from build123d import *

# Parameters (mm, degrees)
SKETCH2_W                      = 38.1
SKETCH2_H                      = 69.85
BOSS_EXTRUDE1_DEPTH            = 4.7625
FILLET1_R                      = 6.35
F_4_CLEARANCE_HOLE1_D          = 2.9464
BOSS_EXTRUDE2_DEPTH            = 9.525
F_8_32_TAPPED_HOLE1_AT_2_COUNT = 2
F_8_32_TAPPED_HOLE1_AT_2_PITCH = 28.575
F_8_32_TAPPED_HOLE1_AT_3_COUNT = 2
F_8_32_TAPPED_HOLE1_AT_3_PITCH = 28.575
SKETCH12_W                     = 19.05
SKETCH12_H                     = 44.45
CUT_EXTRUDE1_DEPTH             = 47.198333888
FILLET2_R                      = 3.175
F_8_32_TAPPED_HOLE2_D          = 3.4544


with BuildPart() as part:
    # Sketch2 → Boss-Extrude1 (new, symmetric)
    with BuildSketch(Plane.XY):
        Rectangle(SKETCH2_W, SKETCH2_H)
    extrude(amount=BOSS_EXTRUDE1_DEPTH, both=True)

    # Fillet1
    fillet1_edges = [part.edges().sort_by_distance(p)[0] for p in [
        (19.05, -34.925, 0),
        (-19.05, -34.925, 0),
        (-19.05, 34.925, 0),
        (19.05, 34.925, 0),
    ]]
    fillet(fillet1_edges, radius=FILLET1_R)

    # #4 Clearance Hole1 (through all)
    with Locations(Plane.XY.offset(4.7625)):
        with Locations((0, 29.21), (-15.24, 27.94), (15.24, 27.94), (-15.24, -27.94), (15.24, -27.94), (-16.51, 17.78), (-16.51, -12.7), (16.51, 17.78), (16.51, -12.7), (0, -29.21)):
            Hole(F_4_CLEARANCE_HOLE1_D / 2)

    # Sketch6 → Boss-Extrude2 (add)
    with BuildSketch(Plane(origin=(0, 0, -4.7625), x_dir=(-1, 0, 0), z_dir=(0, 0, -1))):
        with BuildLine():
            Line((-28.702, -34.925), (-12.7, -34.925))
            ThreePointArc((-12.7, -34.925), (-17.190128061, -33.065128061), (-19.05, -28.575))
            Line((-19.05, -28.575), (-19.05, 28.575))
            ThreePointArc((-19.05, 28.575), (-17.190128061, 33.065128061), (-12.7, 34.925))
            Line((-12.7, 34.925), (-28.702, 34.925))
            Line((-28.702, 34.925), (-28.702, -34.925))
        make_face()
        with BuildLine():
            Line((28.702, -34.925), (28.702, 34.925))
            Line((28.702, 34.925), (12.7, 34.925))
            ThreePointArc((12.7, 34.925), (17.190128061, 33.065128061), (19.05, 28.575))
            Line((19.05, 28.575), (19.05, -28.575))
            ThreePointArc((19.05, -28.575), (17.190128061, -33.065128061), (12.7, -34.925))
            Line((12.7, -34.925), (28.702, -34.925))
        make_face()
    extrude(amount=-BOSS_EXTRUDE2_DEPTH)

    # Sketch11 → #8-32 Tapped Hole1 (revolve, cut)
    with BuildSketch(Plane(origin=(28.702, 0, 0), x_dir=(0, 0, -1), z_dir=(0, 1, 0))):
        Polygon((0, 0), (0, 10.562806461), (1.7272, 9.525), (1.7272, 0), align=None)
    f_8_32_tapped_hole1 = revolve(axis=Axis((35.052, 0, 0), (-1, 0, 0)), mode=Mode.SUBTRACT)

    # #8-32 Tapped Hole1 at 2: #8-32 Tapped Hole1 ×2
    with Locations(*[(0, i * F_8_32_TAPPED_HOLE1_AT_2_PITCH, 0) for i in range(1, F_8_32_TAPPED_HOLE1_AT_2_COUNT)]):
        add(f_8_32_tapped_hole1, mode=Mode.SUBTRACT)

    # #8-32 Tapped Hole1 at 3: #8-32 Tapped Hole1 ×2
    with Locations(*[(0, -i * F_8_32_TAPPED_HOLE1_AT_3_PITCH, 0) for i in range(1, F_8_32_TAPPED_HOLE1_AT_3_COUNT)]):
        add(f_8_32_tapped_hole1, mode=Mode.SUBTRACT)

    # Mirror1: #8-32 Tapped Hole1 across plane
    add(f_8_32_tapped_hole1.mirror(Plane(origin=(0, 0, 0), x_dir=(0, 0, 1), z_dir=(1, 0, 0))), mode=Mode.SUBTRACT)

    # Mirror1 copy 1 sketch → Mirror1 copy 1 (revolve, cut)
    with BuildSketch(Plane(origin=(-28.702, 28.575, 0), x_dir=(0, 0, -1), z_dir=(0, 1, 0))):
        Polygon((0, 0), (0, -10.562806461), (1.7272, -9.525), (1.7272, 0), align=None)
    revolve(axis=Axis((-35.052, 28.575, 0), (-1, 0, 0)), mode=Mode.SUBTRACT)

    # Mirror1 copy 2 sketch → Mirror1 copy 2 (revolve, cut)
    with BuildSketch(Plane(origin=(-28.702, -28.575, 0), x_dir=(0, 0, -1), z_dir=(0, 1, 0))):
        Polygon((0, 0), (0, -10.562806461), (1.7272, -9.525), (1.7272, 0), align=None)
    revolve(axis=Axis((-35.052, -28.575, 0), (-1, 0, 0)), mode=Mode.SUBTRACT)

    # Sketch12 → Cut-Extrude1 (cut, through all)
    with BuildSketch(Plane(origin=(0, 0, -4.7625), x_dir=(-1, 0, 0), z_dir=(0, 0, -1))):
        Rectangle(SKETCH12_W, SKETCH12_H)
    extrude(amount=-CUT_EXTRUDE1_DEPTH, mode=Mode.SUBTRACT)

    # Fillet2
    fillet2_edges = [part.edges().sort_by_distance(p)[0] for p in [
        (-9.525, 22.225, 0),
        (-9.525, -22.225, 0),
        (9.525, -22.225, 0),
        (9.525, 22.225, 0),
    ]]
    fillet(fillet2_edges, radius=FILLET2_R)

    # #8-32 Tapped Hole2 (through all)
    with Locations(Plane(origin=(0, 0, -4.7625), x_dir=(-1, 0, 0), z_dir=(0, 0, -1))):
        with Locations((-17.78, -5.08)):
            Hole(F_8_32_TAPPED_HOLE2_D / 2)


solid = part.part
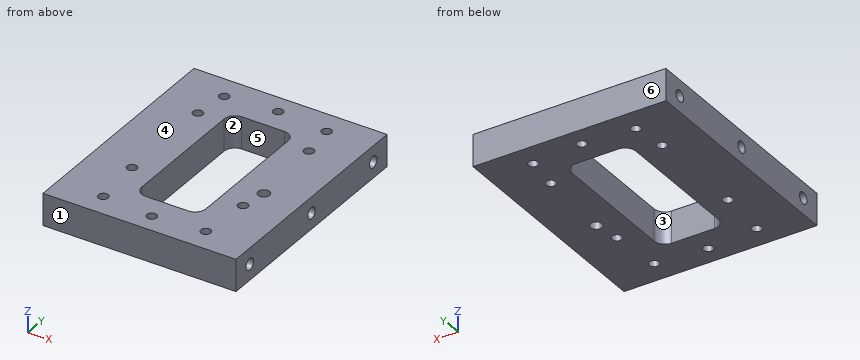
The listing builds one solid part. Answer for the finished solid, in the listing's coordinates (mm). Face numbers are marked on the shaded views. A direction names the side the tool comes from. Give positions to 0.01 mm unless a question says otherwise; leave off trailing zeros. Write each loop counter-clockwise with the first axis right and the second up, starting at its lowest first coordinate (ties: lowest second). Pieces come first, ordered by that corner, then holes. Notation, with made-up numbers: (0, -38) - (32, -38) arc R27 ccw to (32, -4) - close; hole circle Ø6 at (53.25, 60.5). An arc over 180 degrees is marked (long way). One line per question, with ' | ' between items. Start each with the question number.
1. Determine the mould class of the marked faces 3, 4, 5 and 6 for opening direction Y: +Y half, -Y half, draft (parallel to the pull), parting line (faces both ways), or undercut.
2. Section A-A, the plane x = -2.5 is taken. Determine the outline of the cut face in (y, z) (1 decimal), then the cut area to 3 significant figures.
3. Section C-C, the plane z = -3 is taken. Count the separate pieces of the cut face and the enclosed holes in it, then the cut area to 3 significant figures.
4. Given P1, Ø3, axis at y = 28.575, z = 0, coming from the -X side; P2, Ø2.5, axis at x = -15.24, y = 27.94, coming from the -Z side, each flat-ended and moving along its own axis, determine where each tip first touches the part or whether it passes through.
5. Section B-B, the plane y = -9 is taken. Determine the outline of the cut face in (x, z) (1 decimal).
6. For the marked faces 1 and 2, determine the directions among +Z, -Z, +X, -X, +Y, -Y from which every point of the face is accessible in a straight line to the end or side of a thin tool.
7. Straight lines are drawn through the part: line 1 (X direction, y = 0, z = -4) (3 decimals); line 2 (Z direction, x = -24, y = 0); line 3 (Y direction, x = -3.5, z = 2.5) (3 decimals). For each, find the intervals that lie inside material, in ascending order.
Result:
1) face 3: undercut | face 4: draft | face 5: undercut | face 6: +Y half
2) outline: (-34.9, -4.8) - (-22.2, -4.8) - (-22.2, 4.8) - (-34.9, 4.8) - close; (22.2, -4.8) - (34.9, -4.8) - (34.9, 4.8) - (22.2, 4.8) - close | area: 242 mm2
3) separate pieces: 1 | enclosed holes: 12 | area: 3,090 mm2
4) P1: stops at x = -19.04 | P2: passes through
5) outline: (-28.7, -4.8) - (-9.5, -4.8) - (-9.5, 4.8) - (-28.7, 4.8) - close; (9.5, -4.8) - (28.7, -4.8) - (28.7, 4.8) - (9.5, 4.8) - close
6) face 1: +Z, -Z, +X, -X, -Y | face 2: +Z, -Z
7) line 1: x = -28.702 to -9.525, 9.525 to 28.702 | line 2: z = -4.76 to -1.73, 1.73 to 4.76 | line 3: y = -34.925 to -22.225, 22.225 to 34.925
